```python
from build123d import *

# Parameters (mm, degrees)
CROQUIS1_W              = 6.7
CROQUIS1_H              = 6.7
SALIENTE_EXTRUIR1_DEPTH = 80
CROQUIS2_R              = 4.38396011
CORTAR_EXTRUIR1_DEPTH   = 34


with BuildPart() as part:
    # Croquis1 → Saliente-Extruir1 (new body)
    with BuildSketch(Plane.XY):
        with BuildLine():
            Line((-12.05, -30.05), (-4, -30.05))
            Line((-4, -30.05), (-4, -27.75))
            Line((-4, -27.75), (-11.7, -27.75))
            Line((-11.7, -27.75), (-5, -21.05))
            Line((-5, -21.05), (5, -21.05))
            Line((5, -21.05), (11.7, -27.75))
            Line((11.7, -27.75), (4, -27.75))
            Line((4, -27.75), (4, -30.05))
            Line((4, -30.05), (12.05, -30.05))
            ThreePointArc((12.05, -30.05), (14.171320344, -29.171320344), (15.05, -27.05))
            Line((15.05, -27.05), (15.05, -18.55))
            Line((15.05, -18.55), (12.75, -18.55))
            Line((12.75, -18.55), (12.75, -25.8))
            Line((12.75, -25.8), (6.5, -19.55))
            Line((6.5, -19.55), (6.5, -9.55))
            Line((6.5, -9.55), (12.75, -3.3))
            Line((12.75, -3.3), (12.75, -10.55))
            Line((12.75, -10.55), (15.05, -10.55))
            Line((15.05, -10.55), (15.05, 10.55))
            Line((15.05, 10.55), (12.75, 10.55))
            Line((12.75, 10.55), (12.75, 3.3))
            Line((12.75, 3.3), (6.5, 9.55))
            Line((6.5, 9.55), (6.5, 19.55))
            Line((6.5, 19.55), (12.75, 25.8))
            Line((12.75, 25.8), (12.75, 18.55))
            Line((12.75, 18.55), (15.05, 18.55))
            Line((15.05, 18.55), (15.05, 27.05))
            ThreePointArc((15.05, 27.05), (14.171320344, 29.171320344), (12.05, 30.05))
            Line((12.05, 30.05), (4, 30.05))
            Line((4, 30.05), (4, 27.75))
            Line((4, 27.75), (11.7, 27.75))
            Line((11.7, 27.75), (5, 21.05))
            Line((5, 21.05), (-5, 21.05))
            Line((-5, 21.05), (-11.7, 27.75))
            Line((-11.7, 27.75), (-4, 27.75))
            Line((-4, 27.75), (-4, 30.05))
            Line((-4, 30.05), (-12.05, 30.05))
            ThreePointArc((-12.05, 30.05), (-14.171320344, 29.171320344), (-15.05, 27.05))
            Line((-15.05, 27.05), (-15.05, 18.55))
            Line((-15.05, 18.55), (-12.75, 18.55))
            Line((-12.75, 18.55), (-12.75, 25.8))
            Line((-12.75, 25.8), (-6.5, 19.55))
            Line((-6.5, 19.55), (-6.5, 9.55))
            Line((-6.5, 9.55), (-12.75, 3.3))
            Line((-12.75, 3.3), (-12.75, 10.55))
            Line((-12.75, 10.55), (-15.05, 10.55))
            Line((-15.05, 10.55), (-15.05, -10.55))
            Line((-15.05, -10.55), (-12.75, -10.55))
            Line((-12.75, -10.55), (-12.75, -3.3))
            Line((-12.75, -3.3), (-6.5, -9.55))
            Line((-6.5, -9.55), (-6.5, -19.55))
            Line((-6.5, -19.55), (-12.75, -25.8))
            Line((-12.75, -25.8), (-12.75, -18.55))
            Line((-12.75, -18.55), (-15.05, -18.55))
            Line((-15.05, -18.55), (-15.05, -27.05))
            ThreePointArc((-15.05, -27.05), (-14.171320344, -29.171320344), (-12.05, -30.05))
        make_face()
        Polygon((-5, 8.05), (5, 8.05), (11.7, 1.35), (12.75, 0.3), (12.75, -0.3), (11.7, -1.35), (5, -8.05), (-5, -8.05), (-11.7, -1.35), (-12.75, -0.3), (-12.75, 0.3), (-11.7, 1.35), align=None, mode=Mode.SUBTRACT)
        with Locations((0, 14.55)):
            Rectangle(CROQUIS1_W, CROQUIS1_H, mode=Mode.SUBTRACT)
        with Locations((0, -14.55)):
            Rectangle(CROQUIS1_W, CROQUIS1_H, mode=Mode.SUBTRACT)
    extrude(amount=SALIENTE_EXTRUIR1_DEPTH)

    # Croquis2 → Cortar-Extruir1 (cut)
    with BuildSketch(Plane(origin=(15.05, 0, 0), x_dir=(0, 0, -1), z_dir=(1, 0, 0))):
        with Locations((-64.5, 0.3)):
            Circle(CROQUIS2_R)
        with Locations((-15.5, 0.3)):
            Circle(CROQUIS2_R)
    extrude(amount=-CORTAR_EXTRUIR1_DEPTH, mode=Mode.SUBTRACT)


solid = part.part
```
CAD build for the part. Positions are in the model's coordinates, mm. A direction names the side the tool comes from. Round coordinates to 2 decimals unless told otherwise and drop trailing zeros. Order: outer loops, then holes, each group sorted by start corner. A loop starts at its lowest first (then second) coordinate and runs counter-clockwise, first axis right, second up. Notation, with made-up numbers: (-10.75, -33.75) - (35.25, -33.75) arc R9 cw to (35.25, -18.75) - close; hole circle Ø1 at (12, 35.5). An arc over 180 degrees is marked (long way). Use CSV: the item, a comma, the result in double quotes. Start each with the question number.
1) Pin check, flat tips, straight feed: pin 1 Ø1 at (y, z) = (15.5, 67) entering from +X; pin 2 Ø0.7 at (x, z) = (14, 41.5) entering from +Y; pin 3 Ø2 at (x, z) = (-1.5, 58) entering from -Y. Stop position of each tip, or through.
2) Two-plate mould, pull along Y, no slides. Class faces 4 (the flat face through (0, -17.9, 39)), 5 (the flat face through (4, -29, 39)), 6 (the cylindrical face through (-14.19, -29.15, 39.44)), 7 (the flat face through (-12.75, -22, 39)): pulls with the +Y half, pulls with the -Y half, needs draft (parallel to the pull), parting line crosses it, or undercut.
3) Saw through at B-B (z = 15.5). Count the separate pieces of the cut face and the enclosed holes in it, and give its area (3 significant figures).
4) Wall check: L1, parallel to Y at x = -1, z = 64; L2, parallel to Y at x = -7, z = 35; L3, parallel to X at y = -7.5, z = 16. Give the ranges that are in metal, low to high. Write a range as [from, to].
5) Tool access for faces 1 (the cylindrical face through (14.15, -29.19, 39.44)), 2 (the flat face through (0, 21.05, 39)), 3 (the flat face through (-4, -29, 39)): list every direction of +Z, -Z, +X, -X, +Y, -Y with a clear straight run to the whole face (end or side of a thin tool).
6) Saw through at A-A (y = 24). List the corners of the cut face in (x, z), and give its area (3 significant figures).
Values follow:
1,pin 1,"stops at x = 6.5"
1,pin 2,"stops at y = 29.59"
1,pin 3,"stops at y = -21.05"
2,face 4,"undercut"
2,face 5,"needs draft"
2,face 6,"pulls with the -Y half"
2,face 7,"undercut"
3,separate pieces,"6"
3,enclosed holes,"2"
3,area,"609 mm2"
4,L1,"y = [-21.05, -17.9], [-11.2, -8.05], [8.05, 11.2], [17.9, 21.05]"
4,L2,"y = [-30.05, -27.75], [-23.05, -20.05], [-9.05, -6.05], [6.05, 9.05], [20.05, 23.05], [27.75, 30.05]"
4,L3,"x = [-15.05, -12.75], [-8.55, -5.55], [5.55, 8.55], [12.75, 15.05]"
5,face 1,"+Z, -Z, +X, -Y"
5,face 2,"+Z, -Z"
5,face 3,"+Z, -Z, -Y"
6,outline,"(-15.05, 0) - (-12.75, 0) - (-12.75, 80) - (-15.05, 80) - close; (-10.95, 0) - (-7.95, 0) - (-7.95, 80) - (-10.95, 80) - close; (7.95, 0) - (10.95, 0) - (10.95, 80) - (7.95, 80) - close; (12.75, 0) - (15.05, 0) - (15.05, 80) - (12.75, 80) - close"
6,area,"848 mm2"
